from build123d import *

# Parameters (mm, degrees)
ESQUISSE1_R        = 5
BOSS_EXTRU_1_DEPTH = 3


with BuildPart() as part:
    # Esquisse1 → Boss.-Extru.1 (new body)
    with BuildSketch(Plane(origin=(0, 0, 0), x_dir=(1, 0, 0), z_dir=(0, 1, 0))):
        Polygon((-90, 60), (90, 60), (90, 50), (87, 50), (87, 40), (90, 40), (90, 30), (87, 30), (87, 20), (90, 20), (90, 10), (87, 10), (87, 0), (90, 0), (90, -10), (87, -10), (87, -20), (90, -20), (90, -30), (87, -30), (87, -40), (90, -40), (90, -50), (87, -50), (87, -60), (-87, -60), (-87, -50), (-90, -50), (-90, -40), (-87, -40), (-87, -30), (-90, -30), (-90, -20), (-87, -20), (-87, -10), (-90, -10), (-90, 0), (-87, 0), (-87, 10), (-90, 10), (-90, 20), (-87, 20), (-87, 30), (-90, 30), (-90, 40), (-87, 40), (-87, 50), (-90, 50), align=None)
        with Locations((0, -30)):
            Circle(ESQUISSE1_R, mode=Mode.SUBTRACT)
    extrude(amount=BOSS_EXTRU_1_DEPTH)


solid = part.part
Read the model definition and answer for the solid it produces. Units are mm, in the model's axes. Round coordinates to 2 decimals unless told otherwise and drop trailing zeros. Write each loop counter-clockwise with the first axis right and the second up, starting at its lowest first coordinate (ties: lowest second). Pieces come first, ordered by that corner, then holes.
1. Given pin 1 Ø0.9 at (x, y) = (88.5, 1) entering from +Z; pin 2 Ø1.5 at (y, z) = (1.5, 32.5) entering from -X, each flat-ended and moving along its own axis, determine where each tip first touches the part or whether it passes through.
2. Determine the mould class of faces 1 (the face through (1, 3, -1)), 2 (the face through (-1.08, 1.48, 34.88)) for opening direction X: pulls with the +X half, pulls with the -X half, needs draft (parallel to the pull), parting line crosses it, or undercut.
3. The part is cut by section A-A, the plane z = 27. Determine the outline of the cut face in (x, y).
4. The part is cut by section B-B, the plane x = 0. Determine the outline of the cut face in (y, z), then the cut area to 3 significant figures.
5. Straight lines are drawn through the part: L1, parallel to Z at x = 0, y = 1.75; L2, parallel to X at y = 0.6, z = 17; L3, parallel to X at y = 1.35, z = 32.5. For each, find the intervals that lie inside material, in ascending order.
6. The part is cut by section C-C, the plane z = -45. Determine the outline of the cut face in (x, y).
Values:
1. pin 1: stops at z = 50
1. pin 2: stops at x = -87
2. face 1: needs draft
2. face 2: undercut
3. outline: (-90, 0) - (-4, 0) - (-4, 3) - (-90, 3) - close; (4, 0) - (90, 0) - (90, 3) - (4, 3) - close
4. outline: (0, -60) - (3, -60) - (3, 25) - (0, 25) - close; (0, 35) - (3, 35) - (3, 60) - (0, 60) - close
4. area: 330 mm2
5. L1: z = -60 to 25, 35 to 60
5. L2: x = -87 to 87
5. L3: x = -87 to -4.33, 4.33 to 87
6. outline: (-87, 0) - (87, 0) - (87, 3) - (-87, 3) - close
